Could you check a few things on this drawing? It's one solid part, dimensions in mm from its lowest x, y, z. Give positions to 0.01 mm unless a question says otherwise; leave off trailing zeros. Order: outer loops, then holes, each group sorted by start corner. A loop starts at its lowest first (then second) coordinate and runs counter-clockwise, first axis right, second up.
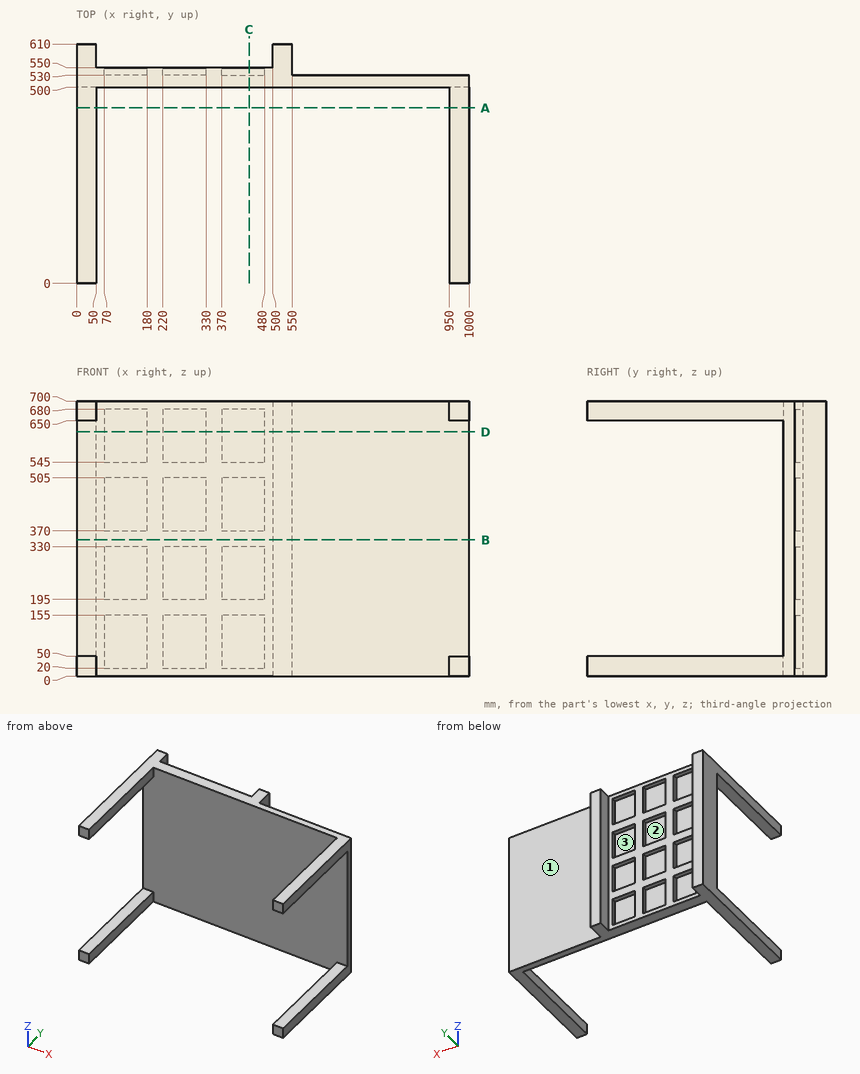
Item 1: We'd pull the mould along X, two halves only. Please class the marked faces 1, 2 and 3: +X half, -X half, draft (parallel to the pull), parting line (faces both ways), or undercut.
Findings:
face 1: draft
face 2: undercut
face 3: undercut
Item 2: For pin 1 (10 mm diameter, centred on x = 623.5, z = 582, fed in from +Y); pin 2 (6 mm diameter, centred on y = 540, z = 293, fed in from +X), each with a flat end and sliding along its axis, tell me the tip position at first contact or that it passes through.
Findings:
pin 1: stops at y = 530
pin 2: stops at x = 550
Item 3: Imagine slicing it at D-D on z = 622. List the corners of the cut face in (x, y) for me.
Findings:
outline: (0, 500) - (1000, 500) - (1000, 530) - (550, 530) - (550, 610) - (500, 610) - (500, 550) - (480, 550) - (480, 530) - (370, 530) - (370, 550) - (330, 550) - (330, 530) - (220, 530) - (220, 550) - (180, 550) - (180, 530) - (70, 530) - (70, 550) - (50, 550) - (50, 610) - (0, 610) - close
Item 4: Imagine slicing it at C-C on x = 439.5. List the corners of the cut face in (y, z) for me, then the cut area to 3 significant figures.
Findings:
outline: (500, 0) - (550, 0) - (550, 20) - (530, 20) - (530, 155) - (550, 155) - (550, 195) - (530, 195) - (530, 330) - (550, 330) - (550, 370) - (530, 370) - (530, 505) - (550, 505) - (550, 545) - (530, 545) - (530, 680) - (550, 680) - (550, 700) - (500, 700) - close
area: 24,200 mm2
Item 5: Imagine slicing it at A-A on y = 447.5. List the corners of the cut face in (x, z) for me, then the cut area to 3 significant figures.
Findings:
outline: (0, 0) - (50, 0) - (50, 50) - (0, 50) - close; (0, 650) - (50, 650) - (50, 700) - (0, 700) - close; (950, 0) - (1000, 0) - (1000, 50) - (950, 50) - close; (950, 650) - (1000, 650) - (1000, 700) - (950, 700) - close
area: 10,000 mm2
Item 6: Please list where these lines run through material, in increasing order: line 1 along X through (y, z) = (167.5, 670); line 2 along Y through (x, z) = (507, 226); line 3 along Y through (x, z) = (220.5, 356.5).
Findings:
line 1: x = 0 to 50, 950 to 1000
line 2: y = 500 to 610
line 3: y = 500 to 550
Item 7: Imagine slicing it at B-B on z = 347. List the corners of the cut face in (x, y) for me.
Findings:
outline: (0, 500) - (1000, 500) - (1000, 530) - (550, 530) - (550, 610) - (500, 610) - (500, 550) - (50, 550) - (50, 610) - (0, 610) - close
